For this review, take the finished solid that the model builds, in its own axes (mm). Face numbers are marked on the shaded views. A direction names the side the tool comes from. Coordinates: 2 decimals unless noted, no trailing zeros. Loops run counter-clockwise (first coordinate to the right, second up) from the corner with the lowest first, then second, coordinate; pieces in that order, holes last. Notation, with made-up numbers: M 37.25,40.25 L 79.25,40.25 A22 ccw 79.25,69.25 Z; hole C 63,25.25 d10. An arc over 180 degrees is marked long. Answer as a JSON object with one key per item and string values. Group by question number.
Item 1: Mouldability with a two-part tool opening along X and no side actions: class the marked faces 4, 5, 6 and 7 as +X half, -X half, draft (parallel to the pull), parting line (faces both ways), or undercut.
Item 2: Wall thickness on L1, parallel to X at y = -7, z = -0.25; L2, parallel to Y at x = 1, z = 6.25 (3 decimals); L3, parallel to X at y = -19.5, z = 4.25: over which ranges is each line inside the solid? List them lowest first. Write a range as from..to.
Item 3: Insertion check: pin 1 (3 mm diameter, centred on x = -4, y = -17, fed in from -Z); pin 2 (2.5 mm diameter, centred on x = 3, z = -2, fed in from -Y) (3 decimals); pin 3 (1 mm diameter, centred on x = 3, y = -17, fed in from +Z). Each pin has a flat end and moves straight along its axis. Give the tip position at first contact, or say it passes through.
Item 4: Add section C-C (x = -3.25). State the section outline as (y, z) points (1 decimal).
Item 5: Tool access review of the marked faces 1, 2 and 3: name each direction out of +Z, -Z, +X, -X, +Y, -Y from which nothing blocks a thin tool from reaching the whole face with its end or side.
from build123d import *

# Parameters (mm, degrees)
F0_R     = 9.525
F1_DEPTH = 25.4
F3_DEPTH = 25.401
F4_DEPTH = 9.525
F6_DEPTH = 9.525


with BuildPart() as f1:
    # F0 (on Front) → F1 (new body)
    with BuildSketch(Plane.XZ):
        Circle(F0_R)
    extrude(amount=F1_DEPTH)

    # F2 (on face) → F3 (cut, through all)
    with BuildSketch(Plane.XZ.offset(25.4)):
        with BuildLine():
            ThreePointArc((-4.7625, 0), (-3.367596, -3.367596), (0, -4.7625))
            ThreePointArc((0, -4.7625), (3.367596, -3.367596), (4.7625, 0))
            ThreePointArc((4.7625, 0), (3.367596, 3.367596), (0, 4.7625))
            ThreePointArc((0, 4.7625), (-3.367596, 3.367596), (-4.7625, 0))
        make_face()
    extrude(amount=-F3_DEPTH, mode=Mode.SUBTRACT)

    # F2 (on face) → F4 (cut)
    with BuildSketch(Plane.XZ.offset(25.4)):
        with BuildLine():
            Line((0, -4.7625), (4.7625, -4.7625))
            Line((4.7625, -4.7625), (4.7625, 0))
            ThreePointArc((4.7625, 0), (3.367596, -3.367596), (0, -4.7625))
        make_face()
        with BuildLine():
            Line((-4.7625, -4.7625), (0, -4.7625))
            ThreePointArc((0, -4.7625), (-3.367596, -3.367596), (-4.7625, 0))
            Line((-4.7625, 0), (-4.7625, -4.7625))
        make_face()
        with BuildLine():
            ThreePointArc((0, 4.7625), (3.367596, 3.367596), (4.7625, 0))
            Line((4.7625, 0), (4.7625, 4.7625))
            Line((4.7625, 4.7625), (0, 4.7625))
        make_face()
        with BuildLine():
            Line((-4.7625, 4.7625), (-4.7625, 0))
            ThreePointArc((-4.7625, 0), (-3.367596, 3.367596), (0, 4.7625))
            Line((0, 4.7625), (-4.7625, 4.7625))
        make_face()
    extrude(amount=-F4_DEPTH, mode=Mode.SUBTRACT)

    # F5 (on Front) → F6 (cut)
    with BuildSketch(Plane.XZ):
        Polygon((6.324151, 3.65125), (0, 7.3025), (-6.324151, 3.65125), (-6.324151, -3.65125), (0, -7.3025), (6.324151, -3.65125), align=None)
    extrude(amount=F6_DEPTH, mode=Mode.SUBTRACT)


solid = f1.part
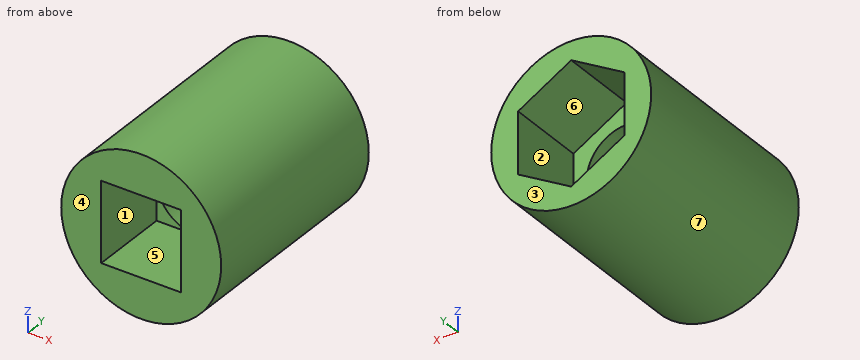
From the geometry:
{
 "1": {"face 4": "draft", "face 5": "undercut", "face 6": "undercut", "face 7": "parting line"},
 "2": {"L1": "x = -9.52..-6.32, 6.32..9.52", "L2": "y = -25.4..-9.525", "L3": "x = -8.52..-4.76, 4.76..8.52"},
 "3": {"pin 1": "stops at z = -9.19", "pin 2": "stops at y = -15.875", "pin 3": "stops at z = 9.19"},
 "4": {"outline": "M -25.4,-9 L 0,-9 L 0,-5.4 L -9.5,-5.4 L -9.5,-3.5 L -15.9,-3.5 L -15.9,-4.8 L -25.4,-4.8 Z; M -25.4,4.8 L -15.9,4.8 L -15.9,3.5 L -9.5,3.5 L -9.5,5.4 L 0,5.4 L 0,9 L -25.4,9 Z"},
 "5": {"face 1": "-Y", "face 2": "+Y", "face 3": "+Z, -Z, +X, -X, +Y"}
}
